Check sheet for the modelled part. Datum: model origin and axes. Units: mm. Coordinates: 2 decimals unless noted, no trailing zeros. Loops run counter-clockwise (first coordinate to the right, second up) from the corner with the lowest first, then second, coordinate; pieces in that order, holes last. Notation, with made-up numbers: M 25,45.5 L 84,45.5 A7 cw 84,55.5 Z; hole C 16,30.25 d1. An arc over 180 degrees is marked long. Use CSV: the item, a comma, the result in double quotes. Start each with the question number.
(1) Scan lines: line 1 (X direction, y = -42, z = 0); line 2 (X direction, y = -276.5, z = 0.95); line 3 (X direction, y = -168, z = -0.05). Record each from-to range of solid material in increasing order.
(2) Section check B-B on z = -1.05. Give the number of separate pieces and of enclosed holes in the cut face, and give its area (3 significant figures).
(3) Section check A-A on x = -17.5. Record the cut outline in (y, z).
(4) Go/stop test with flat-tipped pins: pin 1 Ø0.9 at (y, z) = (-342, 0) entering from -X; pin 2 Ø0.9 at (x, z) = (171.5, -0.5) entering from -Y; pin 3 Ø1.5 at (y, z) = (-346.5, -0.5) entering from +X. Record where each tip stops, or that it passes through.
(5) Section check C-C on y = -227. Record the cut outline in (x, z).
from build123d import *

# Parameters (mm, degrees)
SKETCH_1_R              = 3
EXTRUDE_1_DEPTH         = 1.5
SHEET_START             = -1.5
SHEET_METAL_1_OUTLINE_R = 3
SHEET_METAL_1_DEPTH     = 1.5


# Read off the part's stored shape, not the designer's step: Преобразовать-Твердое тело1
with BuildPart() as part:
    # Sketch 1 → Бобышка-Вытянуть1 (new body)
    with BuildSketch(Plane.XY):
        with BuildLine():
            Line((389.31902002, 22), (-389.31902002, 22))
            ThreePointArc((-389.31902002, 22), (-397.979274058, 17), (-397.979274058, 7))
            Line((-397.979274058, 7), (-376.299038106, -30.551270189))
            Line((-376.299038106, -30.551270189), (-392.320508076, -39.801270189))
            Line((-392.320508076, -39.801270189), (-382.320508076, -57.121778265))
            Line((-382.320508076, -57.121778265), (-366.299038106, -47.871778265))
            Line((-366.299038106, -47.871778265), (-241.299038106, -264.378129211))
            Line((-241.299038106, -264.378129211), (-257.320508076, -273.628129211))
            Line((-257.320508076, -273.628129211), (-247.320508076, -290.948637287))
            Line((-247.320508076, -290.948637287), (-231.299038106, -281.698637287))
            Line((-231.299038106, -281.698637287), (-203.75277675, -329.410161514))
            ThreePointArc((-203.75277675, -329.410161514), (-200.092522712, -333.070415552), (-195.092522712, -334.410161514))
            Line((-195.092522712, -334.410161514), (-149.133974596, -334.410161514))
            Line((-149.133974596, -334.410161514), (-149.133974596, -352.910161514))
            Line((-149.133974596, -352.910161514), (-129.133974596, -352.910161514))
            Line((-129.133974596, -352.910161514), (-129.133974596, -334.410161514))
            Line((-129.133974596, -334.410161514), (129.133974596, -334.410161514))
            Line((129.133974596, -334.410161514), (129.133974596, -352.910161514))
            Line((129.133974596, -352.910161514), (149.133974596, -352.910161514))
            Line((149.133974596, -352.910161514), (149.133974596, -334.410161514))
            Line((149.133974596, -334.410161514), (195.092522712, -334.410161514))
            ThreePointArc((195.092522712, -334.410161514), (200.092522712, -333.070415552), (203.75277675, -329.410161514))
            Line((203.75277675, -329.410161514), (231.299038106, -281.698637287))
            Line((231.299038106, -281.698637287), (247.320508076, -290.948637287))
            Line((247.320508076, -290.948637287), (257.320508076, -273.628129211))
            Line((257.320508076, -273.628129211), (241.299038106, -264.378129211))
            Line((241.299038106, -264.378129211), (366.299038106, -47.871778265))
            Line((366.299038106, -47.871778265), (382.320508076, -57.121778265))
            Line((382.320508076, -57.121778265), (392.320508076, -39.801270189))
            Line((392.320508076, -39.801270189), (376.299038106, -30.551270189))
            Line((376.299038106, -30.551270189), (397.979274058, 7))
            ThreePointArc((397.979274058, 7), (397.979274058, 17), (389.31902002, 22))
        make_face()
        with Locations((244.309773091, -277.663383249)):
            Circle(SKETCH_1_R, mode=Mode.SUBTRACT)
        with Locations((379.309773091, -43.836524227)):
            Circle(SKETCH_1_R, mode=Mode.SUBTRACT)
        with Locations((139.133974596, -343.660161514)):
            Circle(SKETCH_1_R, mode=Mode.SUBTRACT)
        with Locations((-139.133974596, -343.660161514)):
            Circle(SKETCH_1_R, mode=Mode.SUBTRACT)
        with Locations((-244.309773091, -277.663383249)):
            Circle(SKETCH_1_R, mode=Mode.SUBTRACT)
        with Locations((-379.309773091, -43.836524227)):
            Circle(SKETCH_1_R, mode=Mode.SUBTRACT)
        with Locations((300, 10)):
            Circle(SKETCH_1_R, mode=Mode.SUBTRACT)
        with Locations((-300, 10)):
            Circle(SKETCH_1_R, mode=Mode.SUBTRACT)
    extrude(amount=EXTRUDE_1_DEPTH)

    # Sheet Metal 1 outline → Sheet Metal 1 (add)
    with BuildSketch(Plane.XY.offset(SHEET_START)):
        with BuildLine():
            Line((-149.133974596, -334.410161514), (-149.133974596, -352.910161514))
            Line((-149.133974596, -352.910161514), (-129.133974596, -352.910161514))
            Line((-129.133974596, -352.910161514), (-129.133974596, -334.410161514))
            Line((-129.133974596, -334.410161514), (129.133974596, -334.410161514))
            Line((129.133974596, -334.410161514), (129.133974596, -352.910161514))
            Line((129.133974596, -352.910161514), (149.133974596, -352.910161514))
            Line((149.133974596, -352.910161514), (149.133974596, -334.410161514))
            Line((149.133974596, -334.410161514), (195.092522712, -334.410161514))
            ThreePointArc((195.092522712, -334.410161514), (200.092522712, -333.070415552), (203.75277675, -329.410161514))
            Line((203.75277675, -329.410161514), (231.299038106, -281.698637287))
            Line((231.299038106, -281.698637287), (247.320508076, -290.948637287))
            Line((247.320508076, -290.948637287), (257.320508076, -273.628129211))
            Line((257.320508076, -273.628129211), (241.299038106, -264.378129211))
            Line((241.299038106, -264.378129211), (366.299038106, -47.871778265))
            Line((366.299038106, -47.871778265), (382.320508076, -57.121778265))
            Line((382.320508076, -57.121778265), (392.320508076, -39.801270189))
            Line((392.320508076, -39.801270189), (376.299038106, -30.551270189))
            Line((376.299038106, -30.551270189), (397.979274058, 7))
            ThreePointArc((397.979274058, 7), (397.979274058, 17), (389.31902002, 22))
            Line((389.31902002, 22), (-389.31902002, 22))
            ThreePointArc((-389.31902002, 22), (-397.979274058, 17), (-397.979274058, 7))
            Line((-397.979274058, 7), (-376.299038106, -30.551270189))
            Line((-376.299038106, -30.551270189), (-392.320508076, -39.801270189))
            Line((-392.320508076, -39.801270189), (-382.320508076, -57.121778265))
            Line((-382.320508076, -57.121778265), (-366.299038106, -47.871778265))
            Line((-366.299038106, -47.871778265), (-241.299038106, -264.378129211))
            Line((-241.299038106, -264.378129211), (-257.320508076, -273.628129211))
            Line((-257.320508076, -273.628129211), (-247.320508076, -290.948637287))
            Line((-247.320508076, -290.948637287), (-231.299038106, -281.698637287))
            Line((-231.299038106, -281.698637287), (-203.75277675, -329.410161514))
            ThreePointArc((-203.75277675, -329.410161514), (-200.092522712, -333.070415552), (-195.092522712, -334.410161514))
            Line((-195.092522712, -334.410161514), (-149.133974596, -334.410161514))
        make_face()
        with Locations((-244.309773091, -277.663383249)):
            Circle(SHEET_METAL_1_OUTLINE_R, mode=Mode.SUBTRACT)
        with Locations((-139.133974596, -343.660161514)):
            Circle(SHEET_METAL_1_OUTLINE_R, mode=Mode.SUBTRACT)
        with Locations((139.133974596, -343.660161514)):
            Circle(SHEET_METAL_1_OUTLINE_R, mode=Mode.SUBTRACT)
        with Locations((244.309773091, -277.663383249)):
            Circle(SHEET_METAL_1_OUTLINE_R, mode=Mode.SUBTRACT)
        with Locations((-379.309773091, -43.836524227)):
            Circle(SHEET_METAL_1_OUTLINE_R, mode=Mode.SUBTRACT)
        with Locations((-300, 10)):
            Circle(SHEET_METAL_1_OUTLINE_R, mode=Mode.SUBTRACT)
        with Locations((379.309773091, -43.836524227)):
            Circle(SHEET_METAL_1_OUTLINE_R, mode=Mode.SUBTRACT)
        with Locations((300, 10)):
            Circle(SHEET_METAL_1_OUTLINE_R, mode=Mode.SUBTRACT)
    extrude(amount=SHEET_METAL_1_DEPTH)


solid = part.part
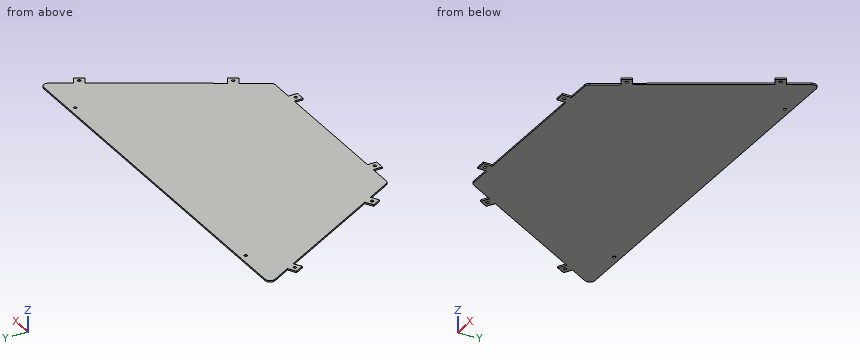
Outcome:
1,line 1,"x = -391.05 to -381.68, -376.94 to 376.94, 381.68 to 391.05"
1,line 2,"x = -255.66 to -247.08, -241.54 to 241.54, 247.08 to 255.66"
1,line 3,"x = -296.94 to 296.94"
2,separate pieces,"1"
2,enclosed holes,"8"
2,area,"218,000 mm²"
3,outline,"M -334.41,-1.5 L 22,-1.5 L 22,1.5 L -334.41,1.5 Z"
4,pin 1,"stops at x = -149.13"
4,pin 2,"stops at y = -334.41"
4,pin 3,"stops at x = 149.13"
5,outline,"M -262.88,-1.5 L 262.88,-1.5 L 262.88,1.5 L -262.88,1.5 Z"
